Build history of the part. All positions in model axes, mm. A direction names the side the tool comes from. Coordinates: 2 decimals unless noted, no trailing zeros. Write each loop counter-clockwise with the first axis right and the second up, starting at its lowest first coordinate (ties: lowest second). Pieces come first, ordered by that corner, then holes. Notation, with made-up numbers: M 89.25,7 L 126.25,7 A22 cw 126.25,21 Z; hole C 48.25,88.5 d3. An arc over 180 degrees is marked long. Use CSV: the item, a comma, the result in double quotes. Start each with the question number.
Autodesk Inventor part; units mm, degrees
ref_plane "YZ Plane" through (0, 0, 0) normal (1, 0, 0) x (0, 1, 0)
ref_plane "XZ Plane" through (0, 0, 0) normal (0, 1, 0) x (-1, 0, 0)
ref_plane "XY Plane" through (0, 0, 0) normal (0, 0, 1) x (1, 0, 0)
sketch "Szkic1" plane through (0, 0, 0) normal (0, 1, 0) x (-1, 0, 0)
  line L0 (-30, 56) -> (30, 56)
  line L1 (30, 56) -> (30, -56)
  line L2 (30, -56) -> (-30, -56)
  line L3 (-30, -56) -> (-30, 56)
  line L4 (-30, 56) -> (30, -56) construction
  line L5 (30, 56) -> (-30, -56) construction
  point P0 (0, 0)
  dimension "d0" = 60
  dimension "d1" = 112
extrude "Płyta1" add sketch "Szkic1" along normal blind 2
sketch "Szkic2" plane through (30, 0, 54) normal (0, 0, 1) x (1, 0, 0)
  line L0 (-60, 0) -> (0, 0)
  line L1 (0, 0) -> (0, 40)
  line L2 (0, 40) -> (-60, 40)
  line L3 (-60, 40) -> (-60, 0)
edge flange "Kołnierz1" height 40 angle 90 thickness 2 bend radius 2.5 thickness toward (0, 0, 1) relief tear relief width 2 relief depth 1 corner gap 2 corner form 0 edges at (0, 2, 56) (0, 2, -56) wall of the first edge with corners at (-30, 0, 54) (30, 0, 54) (30, 40, 54) (-30, 40, 54)
bend "Zagięcie1"
corner "Narożnik1"
sketch "Szkic3" plane through (30, 38, 56) normal (0, 1, 0) x (-1, 0, 0)
  line L0 (60, 0) -> (0, 0)
  line L1 (0, 0) -> (0, -10)
  line L2 (0, -10) -> (60, -10)
  line L3 (60, -10) -> (60, 0)
edge flange "Kołnierz2" height 10 angle 90 thickness 2 bend radius 2.5 thickness toward (0, 1, 0) relief tear relief width 2 relief depth 1 corner gap 2 corner form 0 edges at (0, 40, 54) (0, 40, -54) wall of the first edge with corners at (-30, 38, 56) (30, 38, 56) (30, 38, 46) (-30, 38, 46)
bend "Zagięcie2"
corner "Narożnik2"
sketch "Szkic4" plane through (-30, 40, 46) normal (0, 1, 0) x (1, 0, 0)
  line L0 (60, 92) -> (0, 92)
  line L1 (0, 0) -> (60, 0)
  line L2 (0, 92) -> (0, 97.5)
  line L3 (60, 97.5) -> (60, 92)
  point P0 (30, 46)
  point P1 (8, -2.5)
  point P2 (52, -2.5)
  point P3 (8, 94.5)
  point P4 (52, 94.5)
  dimension "d24" = 2.5
  dimension "d25" = 2.5
  dimension "d26" = 2.5
  dimension "d27" = 2.5
  dimension "d28" = 8
  dimension "d29" = 8
hole "Otwór1" at (-22, 40, 48.5) at (22, 40, 48.5) at (-22, 40, -48.5) at (22, 40, -48.5) direction (0, -1, 0) diameter 2.459 depth 8.8 tip angle 118
sketch "Szkic5" plane through (30, 4.5, -56) normal (0, 0, -1) x (-1, 0, 0)
  line L0 (0, 33.5) -> (0, 31)
  line L1 (0, 32.5) -> (3, 35.5)
  line L2 (0, 35.5) -> (60, 35.5)
  line L3 (0, 35.5) -> (0, 31)
  point P0 (30, -4.5)
  dimension "d37" = 45
  dimension "d38" = 3
extrude "Wyciągnięcie proste1" cut sketch "Szkic5" against normal through all
mirror "Odbij1" about plane through (0, 0, 0) normal (1, 0, 0) of "Wyciągnięcie proste1"
equation "\"d2\" = Grubość"
equation "\"d3\" = SzerokośćGięciaPodcięcia"
equation "\"d4\" = GłębokośćGięciaPodcięcia"
equation "\"d5\" = MinimalnaPozostałość"
equation "\"d6\" = PromieńPrzejścia"
equation "\"d10\" = RozmiarPodcięciaNarożnika"
equation "\"d11\" = Wielk_odstępu"
equation "\"d12\" = Rozmiar_promienia_Jacobiego"
equation "\"d14\" = SzerokośćGięciaPodcięcia"
equation "\"d15\" = GłębokośćGięciaPodcięcia"
equation "\"d16\" = MinimalnaPozostałość"
equation "\"d17\" = PromieńPrzejścia"
equation "\"d21\" = RozmiarPodcięciaNarożnika"
equation "\"d22\" = Wielk_odstępu"
equation "\"d23\" = Rozmiar_promienia_Jacobiego"
equation "\"PromieńGięcia\" = Grubość"
equation "\"SzerokośćGięciaPodcięcia\" = Grubość"
equation "\"GłębokośćGięciaPodcięcia\" = 0.5 * Grubość"
equation "\"RozmiarPodcięciaNarożnika\" = 4 * Grubość"
equation "\"MinimalnaPozostałość\" = 2 * Grubość"
equation "\"PromieńPrzejścia\" = PromieńGięcia"
equation "\"Rozmiar_promienia_Jacobiego\" = PromieńGięcia"
equation "\"Wielk_odstępu\" = Grubość"
properties part number "puszka" material "Stal"
1. Flat gauge pins, fed straight in: pin 1 (18 mm diameter, centred on x = -2, z = 10.5, fed in from +Y); pin 2 (2 mm diameter, centred on x = 22, z = -48.5, fed in from -Y); pin 3 (1 mm diameter, centred on x = -8.5, y = 39, fed in from -Z); pin 4 (2 mm diameter, centred on x = -5.5, y = 39, fed in from +Z). Where does each tip first touch, or does it go through?
2. Slice it at B-B (y = 7.5). List the corners of the cut face in (x, z), and give its area (3 significant figures).
3. Pull direction Y, two halves, no side cores. Call faces 1 (the cylindrical face through (-0.42, 38.717, -54.647)), 2 (the cylindrical face through (-0.42, 37.287, -53.248)), 3 (the cylindrical face through (-20.8, 38.99, 48.23)), 4 (the cylindrical face through (-0.42, 1.353, -54.717)): pulls with the +Y half, pulls with the -Y half, needs draft (parallel to the pull), parting line crosses it, or undercut.
4. Drill centre lines: line 1 along Y through (x, z) = (-9, 47); line 2 along Z through (x, y) = (17, 27.5); line 3 along Z through (x, y) = (22, 38.4). Where is each one in solid material? Low to high. Write a range as from..to.
5. Slice it at C-C (z = 48.5). List the corners of the cut face in (x, y).
6. 3-axis set-ups, long thin cutter, end or side, ignore diameter. For faces 5 (the cylindrical face through (0.42, 2.752, 53.287)), 6 (the cylindrical face through (-20.8, 38.99, -48.77)), 7 (the flat face through (0, 40, 49)): which of +Z, -Z, +X, -X, +Y, -Y reach the whole face in a straight line?
7. Slice it at A-A (x = 22). List the corners of the cut face in (y, z).
8. Slice it at D-D (x = -15.5). List the corners of the cut face in (y, z).
Established:
1,pin 1,"stops at y = 2"
1,pin 2,"stops at y = 0"
1,pin 3,"stops at z = -54.85"
1,pin 4,"stops at z = 55.24"
2,outline,"M -30,-56 L 30,-56 L 30,-54 L -30,-54 Z; M -30,54 L 30,54 L 30,56 L -30,56 Z"
2,area,"240 mm2"
3,face 1,"pulls with the +Y half"
3,face 2,"undercut"
3,face 3,"needs draft"
3,face 4,"pulls with the -Y half"
4,line 1,"y = 0..2, 38..40"
4,line 2,"z = -56..-54, 54..56"
4,line 3,"z = -54.94..-49.73, -47.27..-46, 46..47.27, 49.73..54.94"
5,outline,"M -30,0 L 30,0 L 30,2 L -30,2 Z; M -29,38 L -23.23,38 L -23.23,40 L -27,40 Z; M -20.77,38 L 20.77,38 L 20.77,40 L -20.77,40 Z; M 23.23,38 L 29,38 L 27,40 L 23.23,40 Z"
6,face 5,"+X, -X"
6,face 6,"+Y"
6,face 7,"+Z, -Z, +X, -X, +Y"
7,outline,"M 0,-51.5 A4.5 ccw 4.5,-56 L 35.5,-56 A4.5 ccw 40,-51.5 L 40,-49.73 L 38,-49.73 L 38,-51.5 A2.5 cw 35.5,-54 L 4.5,-54 A2.5 cw 2,-51.5 L 2,51.5 A2.5 cw 4.5,54 L 35.5,54 A2.5 cw 38,51.5 L 38,49.73 L 40,49.73 L 40,51.5 A4.5 ccw 35.5,56 L 4.5,56 A4.5 ccw 0,51.5 Z; M 38,-47.27 L 40,-47.27 L 40,-46 L 38,-46 Z; M 38,46 L 40,46 L 40,47.27 L 38,47.27 Z"
8,outline,"M 0,-51.5 A4.5 ccw 4.5,-56 L 35.5,-56 A4.5 ccw 40,-51.5 L 40,-46 L 38,-46 L 38,-51.5 A2.5 cw 35.5,-54 L 4.5,-54 A2.5 cw 2,-51.5 L 2,51.5 A2.5 cw 4.5,54 L 35.5,54 A2.5 cw 38,51.5 L 38,46 L 40,46 L 40,51.5 A4.5 ccw 35.5,56 L 4.5,56 A4.5 ccw 0,51.5 Z"
